Autodesk Inventor part; units mm, degrees
ref_plane "YZ Plane" through (0, 0, 0) normal (1, 0, 0) x (0, 1, 0)
ref_plane "XZ Plane" through (0, 0, 0) normal (0, 1, 0) x (-1, 0, 0)
ref_plane "XY Plane" through (0, 0, 0) normal (0, 0, 1) x (1, 0, 0)
sketch "Sketch1" plane through (0, 0, 0) normal (0, 0, 1) x (1, 0, 0)
  line L0 (-12.5, 12.5) -> (12.5, 12.5)
  line L1 (27.5, 12.5) -> (27.5, -12.5)
  line L2 (12.5, -12.5) -> (-12.5, -12.5)
  line L3 (-12.5, -12.5) -> (-12.5, 12.5)
  line L4 (-12.5, 12.5) -> (12.5, -12.5) construction
  line L5 (12.5, 12.5) -> (-12.5, -12.5) construction
  line L6 (12.5, 12.5) -> (12.5, -12.5) construction
  line L7 (12.5, 12.5) -> (27.5, 12.5)
  line L8 (12.5, -12.5) -> (27.5, -12.5)
  point P0 (0, 0)
  point P1 (0, 0)
  dimension "d0" = 25
  dimension "d1" = 15
extrude "Extrusion1" add sketch "Sketch1" along normal mid plane 8
sketch "Sketch2" plane through (0, 0, 4) normal (0, 0, 1) x (1, 0, 0)
  point P0 (0, 0)
hole "Hole1" at (0, 0, 4) direction (0, 0, -1) diameter 8.1 end through all
properties part number "BoltRelease" material "ABS Plastic"
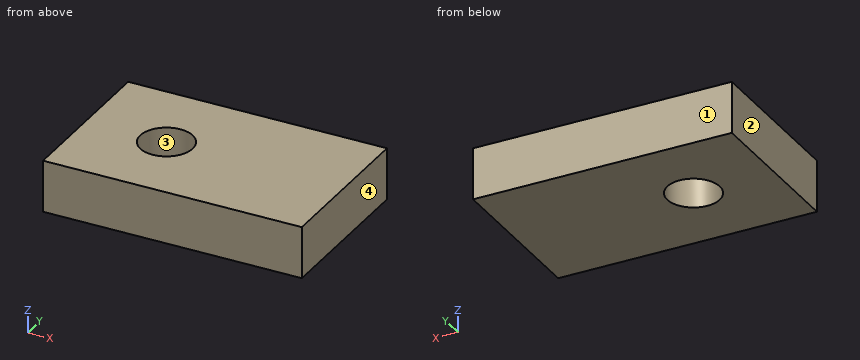
Build history of the part. All positions in model axes, mm. Face numbers are marked on the shaded views. Round coordinates to 2 decimals unless told otherwise and drop trailing zeros. Loops run counter-clockwise (first coordinate to the right, second up) from the corner with the lowest first, then second, coordinate; pieces in that order, holes last. Notation, with made-up numbers: (80.5, 19) -> (89.5, 19) arc R12 cw to (89.5, 32) -> close; hole circle Ø3 at (69.5, 54). An arc over 180 degrees is marked (long way). Answer in a Markdown table with one row per item.
Item 1: Drill centre lines: L1, parallel to X at y = 0, z = -1.75; L2, parallel to Y at x = 0, z = 2.25; L3, parallel to X at y = -1.25, z = -3. Where is each one in solid material? Low to high. Write a range as [from, to].
Answers below:
| item | result |
|---|---|
| L1 | x = [-12.5, -4.05], [4.05, 27.5] |
| L2 | y = [-12.5, -4.05], [4.05, 12.5] |
| L3 | x = [-12.5, -3.85], [3.85, 27.5] |
Item 2: Saw through at B-B (x = 0). Write the cut outline in (y, z), and give its area (3 significant figures).
Answers below:
| item | result |
|---|---|
| outline | (-12.5, -4) -> (-4.05, -4) -> (-4.05, 4) -> (-12.5, 4) -> close; (4.05, -4) -> (12.5, -4) -> (12.5, 4) -> (4.05, 4) -> close |
| area | 135 mm² |
Item 3: Mould opens along X. For the marked faces 1, 2, 3 and 4 say: +X half, -X half, draft (parallel to the pull), parting line (faces both ways), or undercut.
Answers below:
| item | result |
|---|---|
| face 1 | draft |
| face 2 | -X half |
| face 3 | undercut |
| face 4 | +X half |
Item 4: Saw through at C-C (z = 0). Write the cut outline in (x, y).
Answers below:
| item | result |
|---|---|
| outline | (-12.5, -12.5) -> (27.5, -12.5) -> (27.5, 12.5) -> (-12.5, 12.5) -> close; hole circle Ø8.1 at (0, 0) |
Item 5: Saw through at A-A (y = 0). Write the cut outline in (x, z).
Answers below:
| item | result |
|---|---|
| outline | (-12.5, -4) -> (-4.05, -4) -> (-4.05, 4) -> (-12.5, 4) -> close; (4.05, -4) -> (27.5, -4) -> (27.5, 4) -> (4.05, 4) -> close |
